```python
from build123d import *

# Parameters (mm, degrees)
SKETCH1_W           = 20
SKETCH1_H           = 10
SKETCH1_R           = 1.59
SKETCH1_W_2         = 6
SKETCH1_W_3         = 5
BOSS_EXTRUDE1_DEPTH = 3.175
FILLET1_R           = 1


with BuildPart() as part:
    # Sketch1 → Boss-Extrude1 (new body)
    # profile 1 of 3: a face of its own
    with BuildSketch(Plane(origin=(0, 0, 0), x_dir=(1, 0, 0), z_dir=(0, 1, 0))):
        with Locations((6.35, 0)):
            Rectangle(SKETCH1_W, SKETCH1_H)
        with Locations(Location((0, 0, 0), (0, 0, 270))):
            Circle(SKETCH1_R, mode=Mode.SUBTRACT)
        with Locations(Location((12.7, 0, 0), (0, 0, 270))):
            Circle(SKETCH1_R, mode=Mode.SUBTRACT)
    # profile 2 of 3: a face of its own
    with BuildSketch(Plane(origin=(0, 0, 0), x_dir=(1, 0, 0), z_dir=(0, 1, 0))):
        with Locations((-6.65, 0)):
            Rectangle(SKETCH1_W_2, SKETCH1_H)
    # profile 3 of 3: a face of its own
    with BuildSketch(Plane(origin=(0, 0, 0), x_dir=(1, 0, 0), z_dir=(0, 1, 0))):
        with Locations((18.85, 0)):
            Rectangle(SKETCH1_W_3, SKETCH1_H)
    extrude(amount=BOSS_EXTRUDE1_DEPTH)

    # Fillet1
    fillet1_edges = [part.edges().sort_by_distance(p)[0] for p in [
        (-9.65, 1.5875, 5),
        (-9.65, 1.5875, -5),
        (21.35, 1.5875, -5),
        (21.35, 1.5875, 5),
    ]]
    fillet(fillet1_edges, radius=FILLET1_R)


solid = part.part
```
For this review, take the finished solid that the model builds, in its own axes (mm). Coordinates: 2 decimals unless noted, no trailing zeros. Write each loop counter-clockwise with the first axis right and the second up, starting at its lowest first coordinate (ties: lowest second). Pieces come first, ordered by that corner, then holes. Notation, with made-up numbers: (75, -29.5) - (100, -29.5) arc R16 ccw to (100, -21.5) - close; hole circle Ø8 at (80, 8). An arc over 180 degrees is marked (long way). Put each result on its own line as item: value.
1. For pin 1 (3 mm diameter, centred on x = 12.7, z = 0, fed in from -Y), flat-tipped, find the tip position at first contact; note if it passes through.
Values found:
pin 1: through
2. Add section C-C, the plane x = 0. Give the boundary of the cut face in (y, z) (3 decimals).
Values found:
outline: (0, -5) - (3.175, -5) - (3.175, -1.59) - (0, -1.59) - close; (0, 1.59) - (3.175, 1.59) - (3.175, 5) - (0, 5) - close
3. Mouldability with a two-part tool opening along Z and no side actions: class faces 1 (the flat face through (6, 2, -5)), 2 (the flat face through (-9.65, 2, 0)), 3 (the cylindrical face through (14.276, 1.565, -0.207)), 4 (the cylindrical face through (-1.552, 1.565, -0.345)) as released by +Z, released by -Z, zero draft, split by the parting line, or undercut.
Values found:
face 1: released by -Z
face 2: zero draft
face 3: undercut
face 4: undercut
4. Add section A-A, the plane z = 0. Give the boundary of the cut face in (x, y) (3 decimals).
Values found:
outline: (-9.65, 0) - (-1.59, 0) - (-1.59, 3.175) - (-9.65, 3.175) - close; (1.59, 0) - (11.11, 0) - (11.11, 3.175) - (1.59, 3.175) - close; (14.29, 0) - (21.35, 0) - (21.35, 3.175) - (14.29, 3.175) - close
5. Add section B-B, the plane y = 1.75. Give the boundary of the cut face in (x, z).
Values found:
outline: (-9.65, -4) arc R1 ccw to (-8.65, -5) - (20.35, -5) arc R1 ccw to (21.35, -4) - (21.35, 4) arc R1 ccw to (20.35, 5) - (-8.65, 5) arc R1 ccw to (-9.65, 4) - close; hole circle Ø3.18 at (0, 0); hole circle Ø3.18 at (12.7, 0)
6. Wall thickness on probe 1 along X at (y, z) = (0.9, 0); probe 2 along X at (y, z) = (0.7, -1); probe 3 along Z at (x, y) = (11.5, 1.85): over which ranges is each line inside the solid? List them lowest first.
Values found:
probe 1: -9.65 to -1.59, 1.59 to 11.11, 14.29 to 21.35
probe 2: -9.65 to -1.24, 1.24 to 11.46, 13.94 to 21.35
probe 3: -5 to -1.04, 1.04 to 5
